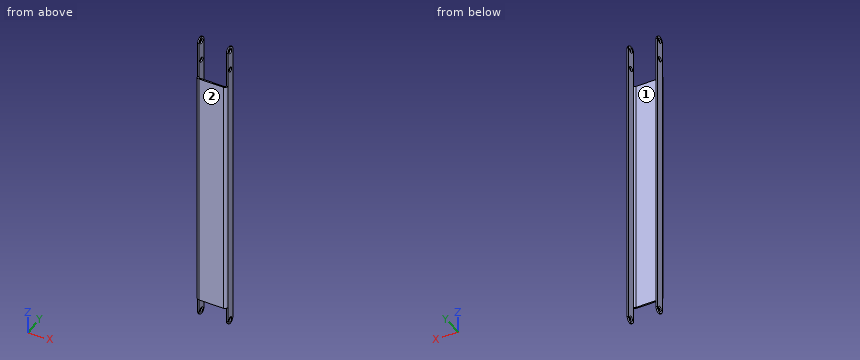
```python
from build123d import *

# Parameters (mm, degrees)
F1_DEPTH = 304.8
F2_R     = 3.69316
F3_R     = 1.98374
F4_W     = 1.70942
F4_H     = 50.8
F4_H_2   = 25.4
F6_DEPTH = 11.1125
F7_R     = 5.55624
F8_R     = 3.175
F9_DEPTH = 38.36416


# Not quite as in the source:
# - a fillet or chamfer is up to 0.001 mm smaller than in the source, because OpenCascade refuses the exact size


with BuildPart() as f1:
    # F0 (on Top) → F1 (new body)
    with BuildSketch(Plane.XY):
        Polygon((0, 13.09624), (0, 0), (-34.94532, 0), (-34.94532, 13.09624), (-36.65474, 13.09624), (-36.65474, -1.70942), (1.70942, -1.70942), (1.70942, 13.09624), align=None)
    extrude(amount=F1_DEPTH)

    # F2
    f2_edges = [f1.edges().sort_by_distance(p)[0] for p in [
        (1.70942, -1.70942, 152.4),
        (-36.65474, -1.70942, 152.4),
    ]]
    fillet(f2_edges, radius=F2_R)

    # F3
    f3_edges = [f1.edges().sort_by_distance(p)[0] for p in [
        (0, 0, 152.4),
        (-34.94532, 0, 152.4),
    ]]
    fillet(f3_edges, radius=F3_R)

    # F4 (on face) → F6 (join, through all)
    with BuildSketch(Plane(origin=(0, 13.09624, 0), x_dir=(-1, 0, 0), z_dir=(0, 1, 0))):
        with Locations((35.80003, 330.2)):
            Rectangle(F4_W, F4_H)
        with Locations((-0.85471, 330.2)):
            Rectangle(F4_W, F4_H)
        with Locations((-0.85471, -12.7)):
            Rectangle(F4_W, F4_H_2)
        with Locations((35.80003, -12.7)):
            Rectangle(F4_W, F4_H_2)
    extrude(amount=-F6_DEPTH)

    # F7 (radius 5.55625 in the source; OpenCascade refuses exactly that, so slightly less here)
    f7_edges = [f1.edges().sort_by_distance(p)[0] for p in [
        (-35.80003, 13.09624, -25.4),
        (0.85471, 13.09624, -25.4),
        (0.85471, 13.09624, 355.6),
        (-35.80003, 13.09624, 355.6),
        (-35.80003, 1.98374, -25.4),
        (-35.80003, 1.98374, 355.6),
        (0.85471, 1.98374, 355.6),
        (0.85471, 1.98374, -25.4),
    ]]
    fillet(f7_edges, radius=F7_R)

    # F8 (on face) → F9 (cut, through all)
    with BuildSketch(Plane.YZ.offset(1.70942)):
        with Locations((7.53999, -19.84375)):
            Circle(F8_R)
        with Locations((7.53999, 350.04375)):
            Circle(F8_R)
        with Locations((7.53999, 324.64375)):
            Circle(F8_R)
    extrude(amount=-F9_DEPTH, mode=Mode.SUBTRACT)


solid = f1.part
```
Input: part model. Units: mm. Frame: model coordinates. Face numbers are marked on the shaded views. Coordinates: 2 decimals unless noted, no trailing zeros. Write each loop counter-clockwise with the first axis right and the second up, starting at its lowest first coordinate (ties: lowest second). Pieces come first, ordered by that corner, then holes.
1) Material intervals for line 1 along X through (y, z) = (7.75, 318.5); line 2 along Y through (x, z) = (-11, 261.5); line 3 along X through (y, z) = (1.5, 56.5), sorted ascending.
2) Section A-A on z = 137. Output: boundary loops of the cut face in (x, y).
3) Section B-B on x = -16.5. Output: boundary loops of the cut face in (y, z), and give its area (3 significant figures).
4) Pin query (flat end, axial travel): pin 1 Ø5.5 at (y, z) = (7.54, 324.64) entering from -X; pin 2 Ø6 at (x, y) = (-8, 0) entering from +Z; pin 3 Ø1.9 at (x, z) = (1, 318) entering from -Y; pin 4 Ø5 at (x, z) = (-3, 305) entering from -Y. Return the tip coordinate at first contact, or that it passes through.
5) Mould query, pull axis X, two halves, no side actions, for the marked faces 1 and 2. Classes: pulls with the +X half, pulls with the -X half, needs draft (parallel to the pull), parting line crosses it, or undercut.
Check result:
1. line 1: x = -36.65 to -34.95, 0 to 1.71
1. line 2: y = -1.71 to 0
1. line 3: x = -36.62 to -34.89, -0.06 to 1.68
2. outline: (-36.65, 1.98) arc R3.69 ccw to (-32.96, -1.71) - (-1.98, -1.71) arc R3.69 ccw to (1.71, 1.98) - (1.71, 13.1) - (0, 13.1) - (0, 1.98) arc R1.98 cw to (-1.98, 0) - (-32.96, 0) arc R1.98 cw to (-34.95, 1.98) - (-34.95, 13.1) - (-36.65, 13.1) - close
3. outline: (-1.71, 0) - (0, 0) - (0, 304.8) - (-1.71, 304.8) - close
3. area: 521 mm2
4. pin 1: passes through
4. pin 2: stops at z = 304.8
4. pin 3: stops at y = 1.98
4. pin 4: stops at y = -1.71
5. face 1: undercut
5. face 2: needs draft
